from build123d import *

# Parameters (mm, degrees)
SKETCH_W        = 90
SKETCH_H        = 76
PAD_DEPTH       = 6
FILLET_R        = 5
SKETCH001_R     = 1.6
POCKET_DEPTH    = 6
SKETCH002_W     = 8
SKETCH002_H     = 15
PAD001_DEPTH    = 8
POCKET001_DEPTH = 90.001
FILLET001_R     = 2


with BuildPart() as part:
    # Sketch → Pad (new body)
    with BuildSketch(Plane.XY):
        Rectangle(SKETCH_W, SKETCH_H)
        with BuildLine():
            ThreePointArc((-34.45, 33), (-37, 35.55), (-39.55, 33))
            Line((-39.55, 33), (-39.55, 28))
            ThreePointArc((-39.55, 28), (-37, 25.45), (-34.45, 28))
            Line((-34.45, 33), (-34.45, 28))
        make_face(mode=Mode.SUBTRACT)
        with BuildLine():
            ThreePointArc((2.55, 33), (0, 35.55), (-2.55, 33))
            Line((-2.55, 33), (-2.55, 28))
            ThreePointArc((-2.55, 28), (0, 25.45), (2.55, 28))
            Line((2.55, 33), (2.55, 28))
        make_face(mode=Mode.SUBTRACT)
        with BuildLine():
            ThreePointArc((39.55, -28), (37, -25.45), (34.45, -28))
            Line((34.45, -28), (34.45, -33))
            ThreePointArc((34.45, -33), (37, -35.55), (39.55, -33))
            Line((39.55, -28), (39.55, -33))
        make_face(mode=Mode.SUBTRACT)
        with BuildLine():
            ThreePointArc((2.55, -28), (0, -25.45), (-2.55, -28))
            Line((-2.55, -28), (-2.55, -33))
            ThreePointArc((-2.55, -33), (0, -35.55), (2.55, -33))
            Line((2.55, -28), (2.55, -33))
        make_face(mode=Mode.SUBTRACT)
        with BuildLine():
            ThreePointArc((-34.45, -28), (-37, -25.45), (-39.55, -28))
            Line((-39.55, -28), (-39.55, -33))
            ThreePointArc((-39.55, -33), (-37, -35.55), (-34.45, -33))
            Line((-34.45, -28), (-34.45, -33))
        make_face(mode=Mode.SUBTRACT)
        with BuildLine():
            ThreePointArc((39.55, 33), (37, 35.55), (34.45, 33))
            Line((34.45, 33), (34.45, 28))
            ThreePointArc((34.45, 28), (37, 25.45), (39.55, 28))
            Line((39.55, 33), (39.55, 28))
        make_face(mode=Mode.SUBTRACT)
    extrude(amount=PAD_DEPTH)

    # Fillet
    fillet_edges = [part.edges().sort_by_distance(p)[0] for p in [
        (45, -38, 3),
        (-45, -38, 3),
        (45, 38, 3),
        (-45, 38, 3),
    ]]
    fillet(fillet_edges, radius=FILLET_R)

    # Sketch001 (on Face5 of Fillet) → Pocket (cut)
    with BuildSketch(Plane.XY.offset(6)):
        with Locations((25, 25)):
            Circle(SKETCH001_R)
        with Locations((25, -25)):
            Circle(SKETCH001_R)
        with Locations((-25, 25)):
            Circle(SKETCH001_R)
        with Locations((-25, -25)):
            Circle(SKETCH001_R)
    extrude(amount=-POCKET_DEPTH, mode=Mode.SUBTRACT)

    # Sketch002 (on Face5 of Pocket) → Pad001 (join)
    with BuildSketch(Plane.XY.offset(6)):
        with Locations((-41, 0)):
            Rectangle(SKETCH002_W, SKETCH002_H)
        with Locations((41, 0)):
            Rectangle(SKETCH002_W, SKETCH002_H)
    extrude(amount=PAD001_DEPTH)

    # Sketch003 (on Face6 of Pad001) → Pocket001 (cut, through all)
    with BuildSketch(Plane(origin=(-45, 0, 0), x_dir=(0, -1, 0), z_dir=(-1, 0, 0))):
        with BuildLine():
            ThreePointArc((-3.5, 11.5), (-5, 10), (-3.5, 8.5))
            Line((-3.5, 8.5), (3.5, 8.5))
            ThreePointArc((3.5, 8.5), (5, 10), (3.5, 11.5))
            Line((-3.5, 11.5), (3.5, 11.5))
        make_face()
    extrude(amount=-POCKET001_DEPTH, mode=Mode.SUBTRACT)

    # Fillet001
    fillet001_edges = [part.edges().sort_by_distance(p)[0] for p in [
        (-41, 7.5, 14),
        (-41, -7.5, 14),
        (41, -7.5, 14),
        (41, 7.5, 14),
    ]]
    fillet(fillet001_edges, radius=FILLET001_R)


solid = part.part
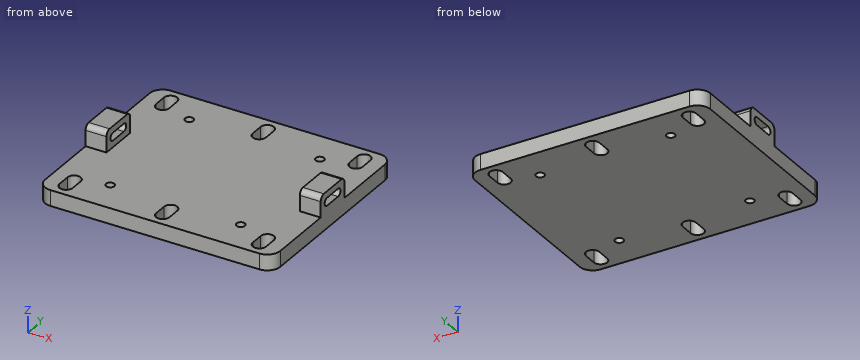
Here's how the part is built. I have some questions about the finished solid (model axes, mm). Round coordinates to 2 decimals unless told otherwise and drop trailing zeros. Loops run counter-clockwise (first coordinate to the right, second up) from the corner with the lowest first, then second, coordinate; pieces in that order, holes last. Notation, with made-up numbers: (37.25, 19) - (86.25, 19) arc R20 cw to (86.25, 55) - close; hole circle Ø10 at (-7, 75). An arc over 180 degrees is marked (long way). One line per question, with ' | ' between items. Start each with the question number.
Q1. Please list where these lines run through material, in increasing order: line 1 (Y direction, x = -25, z = 4.2); line 2 (X direction, y = 33.5, z = 2.5); line 3 (Y direction, x = 1, z = 2.75). Write a range as [from, to].
Q2. I want a section at D-D (x = 25). Write out the boundary of the cut face in (y, z), then the cut area to 3 significant figures.
Q3. I want a section at C-C (y = 29.5). Write out the boundary of the cut face in (x, z), then the cut area to 3 significant figures.
Q4. I want a section at A-A (x = 0). Write out the boundary of the cut face in (y, z), then the cut area to 3 significant figures.
Q5. Will these pins go through, and if not, where does the flat tip stop? pin 1 (2.5 mm diameter, centred on x = 25, y = -25, fed in from -Z); pin 2 (4 mm diameter, centred on x = -25, y = 25, fed in from +Z); pin 3 (1.8 mm diameter, centred on x = -40, z = 9, fed in from +Y).
Q6. I want a section at B-B (z = 7.25). Write out the boundary of the cut face in (x, y), then the cut area to 3 significant figures.
Response values:
1) line 1: y = [-38, -26.6], [-23.4, 23.4], [26.6, 38] | line 2: x = [-44.97, -39.5], [-34.5, -2.5], [2.5, 34.5], [39.5, 44.97] | line 3: y = [-38, -35.35], [-25.65, 25.65], [35.35, 38]
2) outline: (-38, 0) - (-26.6, 0) - (-26.6, 6) - (-38, 6) - close; (-23.4, 0) - (23.4, 0) - (23.4, 6) - (-23.4, 6) - close; (26.6, 0) - (38, 0) - (38, 6) - (26.6, 6) - close | area: 418 mm²
3) outline: (-45, 0) - (-39.55, 0) - (-39.55, 6) - (-45, 6) - close; (-34.45, 0) - (-2.55, 0) - (-2.55, 6) - (-34.45, 6) - close; (2.55, 0) - (34.45, 0) - (34.45, 6) - (2.55, 6) - close; (39.55, 0) - (45, 0) - (45, 6) - (39.55, 6) - close | area: 448 mm²
4) outline: (-38, 0) - (-35.55, 0) - (-35.55, 6) - (-38, 6) - close; (-25.45, 0) - (25.45, 0) - (25.45, 6) - (-25.45, 6) - close; (35.55, 0) - (38, 0) - (38, 6) - (35.55, 6) - close | area: 335 mm²
5) pin 1: passes through | pin 2: stops at z = 6 | pin 3: stops at y = 7.5
6) outline: (-45, -7.5) - (-37, -7.5) - (-37, 7.5) - (-45, 7.5) - close; (37, -7.5) - (45, -7.5) - (45, 7.5) - (37, 7.5) - close | area: 240 mm²
